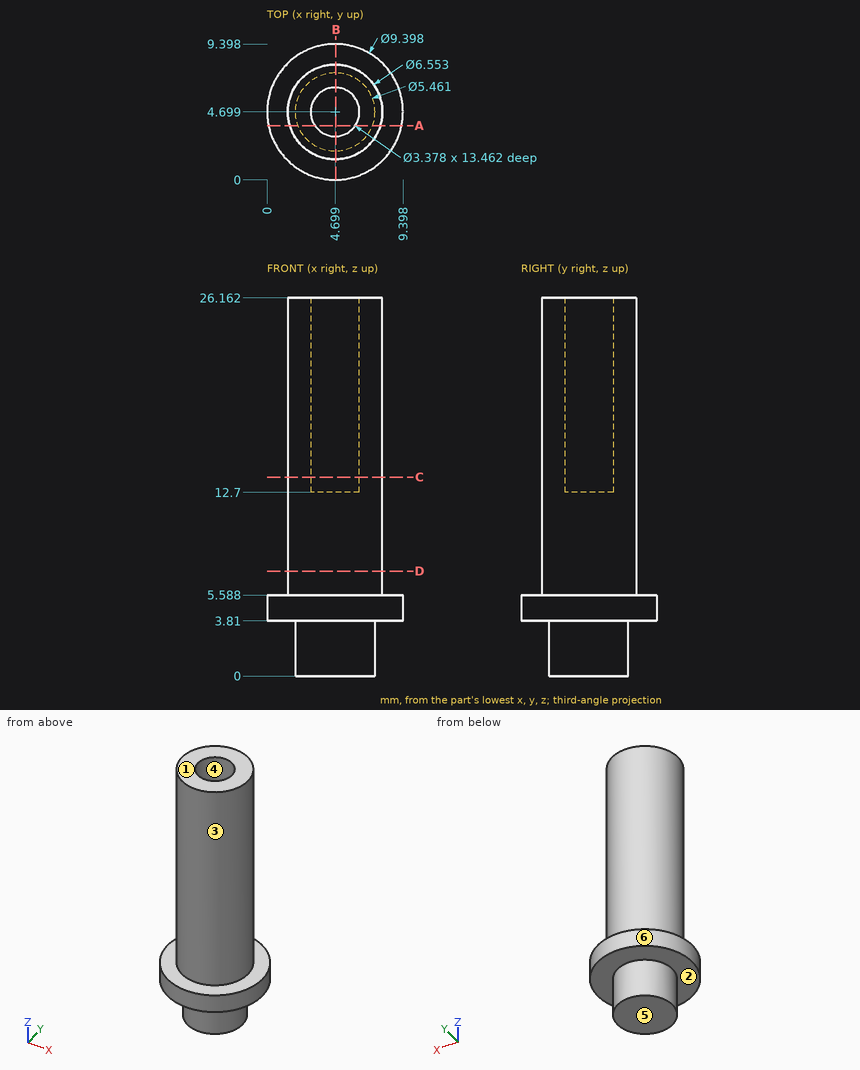
For this review, use the dimensioned drawing (mm, ordinates from the lowest corner) and the shaded views. A direction names the side the tool comes from. Round coordinates to 2 decimals unless told otherwise and drop trailing zeros. Order: outer loops, then holes, each group sorted by start corner. A loop starts at its lowest first (then second) coordinate and runs counter-clockwise, first axis right, second up.
1) Clearance check with flat-ended pins moving along their axes: pin 1 Ø5 at (x, y) = (2, 4) entering from -Z; pin 2 Ø5 at (y, z) = (8, 3.5) entering from +X; pin 3 Ø2 at (x, y) = (4.699, 4.699) entering from +Z. State where each tip first meets the part, or that it passes through.
The answers:
pin 1: stops at z = 0
pin 2: stops at x = 9.33
pin 3: stops at z = 12.7
2) Consider section A-A (y = 3.75). State the section outline as (x, z) points (1 decimal), plus the area to 3 significant figures.
The answers:
outline: (0.1, 3.8) - (2.1, 3.8) - (2.1, 0) - (7.3, 0) - (7.3, 3.8) - (9.3, 3.8) - (9.3, 5.6) - (7.8, 5.6) - (7.8, 26.2) - (6.1, 26.2) - (6.1, 12.7) - (3.3, 12.7) - (3.3, 26.2) - (1.6, 26.2) - (1.6, 5.6) - (0.1, 5.6) - close
area: 127 mm2
3) Consider section C-C (z = 13.75). State the section outline as (x, y) points, plus the area to 3 significant figures.
The answers:
outline: circle Ø6.55 at (4.7, 4.7); hole circle Ø3.38 at (4.7, 4.7)
area: 24.8 mm2
4) For L1, parallel to Z at x = 2, y = 7.5; L2, parallel to X at y = 4.5, z = 7.5; L3, parallel to Y at x = 5.5, z = 16.25, list the stretches that pass through material, from the lowest coordinate up.
The answers:
L1: z = 3.81 to 5.59
L2: x = 1.43 to 7.97
L3: y = 1.52 to 3.21, 6.19 to 7.88
5) Machinability: for the marked faces 1, 2 and 3, which of the approach directions +Z, -Z, +X, -X, +Y, -Y give a long, thin tool a straight path to every point of the face, cutting with its end or side? Answer none if there is none.
The answers:
face 1: +Z, +X, -X, +Y, -Y
face 2: -Z
face 3: +Z
6) Consider section B-B (x = 4.75). State the section outline as (y, z) points (1 decimal).
The answers:
outline: (0, 3.8) - (2, 3.8) - (2, 0) - (7.4, 0) - (7.4, 3.8) - (9.4, 3.8) - (9.4, 5.6) - (8, 5.6) - (8, 26.2) - (6.4, 26.2) - (6.4, 12.7) - (3, 12.7) - (3, 26.2) - (1.4, 26.2) - (1.4, 5.6) - (0, 5.6) - close
7) Draft analysis for pull direction Y (two halves, no side actions). For the marked faces 4, 5 and 6, state which applies: released by +Y, released by -Y, zero draft, split by the parting line, or undercut.
The answers:
face 4: undercut
face 5: zero draft
face 6: split by the parting line
8) Consider section D-D (z = 7.25). State the section outline as (x, y) points.
The answers:
outline: circle Ø6.55 at (4.7, 4.7)
